Geometry: final body of the model. Coordinates: model frame, mm. Give positions to 0.01 mm unless a question says otherwise; leave off trailing zeros. Write each loop counter-clockwise with the first axis right and the second up, starting at its lowest first coordinate (ties: lowest second). Pieces come first, ordered by that corner, then holes. Notation, with made-up numbers: M 63,73.25 L 109,73.25 A19 cw 109,106.25 Z; hole C 69,52.25 d2. An arc over 180 degrees is marked long. Use a Markdown table: item, result. Add a question column.
(1) Material intervals for L1, parallel to Y at x = 2.45, z = -51; L2, parallel to Y at x = 0.7, z = -25.4; L3, parallel to Y at x = 2.2, z = -79, sorted ascending.
(2) Cut plane D-D (y = 71). Output: boundary loops of the cut face in (x, z).
(3) Cut plane A-A (z = -50.8). Output: boundary loops of the cut face in (x, y) (1 decimal).
(4) Cut plane B-B (y = 139.7). Output: boundary loops of the cut face in (x, z).
(5) Cut plane C-C (x = 0.65). State how many separate pieces and enclosed holes the cut face has, plus the area to 3 significant figures.
```python
from build123d import *

# Parameters (mm, degrees)
SKETCH1_W           = 101.6
SKETCH1_H           = 152.4
SKETCH1_R           = 2.54
SKETCH1_R_2         = 13.462
BOSS_EXTRUDE2_DEPTH = 2.54
SKETCH2_R           = 3.4925
CUT_EXTRUDE1_DEPTH  = 184.179615678
LPATTERN2_COUNT     = 2
LPATTERN2_PITCH     = 25.4
LPATTERN3_COUNT     = 2
LPATTERN3_PITCH     = 25.4
FILLET1_R           = 3.175


with BuildPart() as part:
    # Sketch1 → Boss-Extrude2 (new body)
    with BuildSketch(Plane(origin=(0, 0, 0), x_dir=(0, 0, -1), z_dir=(1, 0, 0))):
        with Locations((50.8, 76.2)):
            Rectangle(SKETCH1_W, SKETCH1_H)
        with Locations((78.105, 76.2)):
            Circle(SKETCH1_R, mode=Mode.SUBTRACT)
        with Locations((50.8, 76.2)):
            Circle(SKETCH1_R_2, mode=Mode.SUBTRACT)
        with Locations((50.8, 48.895)):
            Circle(SKETCH1_R, mode=Mode.SUBTRACT)
        with Locations((23.495, 76.2)):
            Circle(SKETCH1_R, mode=Mode.SUBTRACT)
        with Locations((50.8, 103.505)):
            Circle(SKETCH1_R, mode=Mode.SUBTRACT)
    extrude(amount=BOSS_EXTRUDE2_DEPTH)

    # Sketch2 → Cut-Extrude1 (cut, through all)
    with BuildSketch(Plane(origin=(2.54, 0, 0), x_dir=(0, 0, -1), z_dir=(1, 0, 0))):
        with Locations((50.8, 139.7)):
            Circle(SKETCH2_R)
        with Locations((50.8, 12.7)):
            Circle(SKETCH2_R)
    cut_extrude1 = extrude(amount=-CUT_EXTRUDE1_DEPTH, mode=Mode.SUBTRACT)

    # LPattern2: Cut-Extrude1 ×2
    with Locations(*[(0, 0, -i * LPATTERN2_PITCH) for i in range(1, LPATTERN2_COUNT)]):
        add(cut_extrude1, mode=Mode.SUBTRACT)

    # LPattern3: Cut-Extrude1 ×2
    with Locations(*[(0, 0, i * LPATTERN3_PITCH) for i in range(1, LPATTERN3_COUNT)]):
        add(cut_extrude1, mode=Mode.SUBTRACT)

    # Fillet1
    fillet1_edges = [part.edges().sort_by_distance(p)[0] for p in [
        (1.27, 152.4, 0),
        (1.27, 152.4, -101.6),
        (1.27, 0, -101.6),
        (1.27, 0, 0),
    ]]
    fillet(fillet1_edges, radius=FILLET1_R)


solid = part.part
```
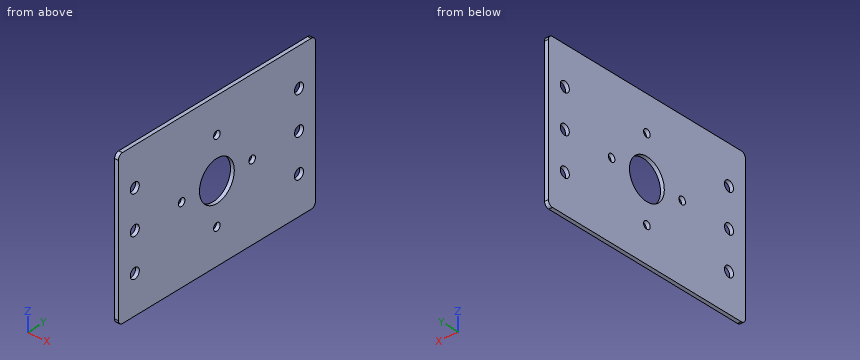
Answer list:
| question | item | result |
|---|---|---|
| 1 | L1 | 0 to 9.21, 16.19 to 46.36, 51.43 to 62.74, 89.66 to 100.97, 106.04 to 136.21, 143.19 to 152.4 |
| 1 | L2 | 0 to 9.21, 16.19 to 74.52, 77.88 to 136.21, 143.19 to 152.4 |
| 1 | L3 | 0 to 10.61, 14.79 to 73.82, 78.58 to 137.61, 141.79 to 152.4 |
| 2 | outline | M 0,-101.6 L 2.54,-101.6 L 2.54,-63.22 L 0,-63.22 Z; M 0,-38.38 L 2.54,-38.38 L 2.54,0 L 0,0 Z |
| 3 | outline | M 0,0 L 2.5,0 L 2.5,9.2 L 0,9.2 Z; M 0,16.2 L 2.5,16.2 L 2.5,46.4 L 0,46.4 Z; M 0,51.4 L 2.5,51.4 L 2.5,62.7 L 0,62.7 Z; M 0,89.7 L 2.5,89.7 L 2.5,101 L 0,101 Z; M 0,106 L 2.5,106 L 2.5,136.2 L 0,136.2 Z; M 0,143.2 L 2.5,143.2 L 2.5,152.4 L 0,152.4 Z |
| 4 | outline | M 0,-101.6 L 2.54,-101.6 L 2.54,-79.69 L 0,-79.69 Z; M 0,-72.71 L 2.54,-72.71 L 2.54,-54.29 L 0,-54.29 Z; M 0,-47.31 L 2.54,-47.31 L 2.54,-28.89 L 0,-28.89 Z; M 0,-21.91 L 2.54,-21.91 L 2.54,0 L 0,0 Z |
| 5 | separate pieces | 1 |
| 5 | enclosed holes | 11 |
| 5 | area | 14,600 mm² |
